Work out the finished part from the listing and answer in its coordinate system (mm). A direction names the side the tool comes from. Coordinates: 2 decimals unless noted, no trailing zeros. Write each loop counter-clockwise with the first axis right and the second up, starting at its lowest first coordinate (ties: lowest second). Pieces come first, ordered by that corner, then holes. Notation, with made-up numbers: (26.25, 10) - (72.25, 10) arc R20 ccw to (72.25, 20) - close; hole circle Ø4 at (60, -5.75). An arc over 180 degrees is marked (long way). One line per item, written item: value.
```python
from build123d import *

# Parameters (mm, degrees)
SKETCH1_R           = 17.35
BOSS_EXTRUDE1_DEPTH = 7
SKETCH2_R           = 31
BOSS_EXTRUDE2_DEPTH = 2
SKETCH3_R           = 14.646692659
CUT_EXTRUDE1_DEPTH  = 7
CHAMFER1_SIZE       = 1


with BuildPart() as part:
    # Sketch1 → Boss-Extrude1 (new body)
    with BuildSketch(Plane(origin=(0, 0, 0), x_dir=(1, 0, 0), z_dir=(0, 1, 0))):
        Circle(SKETCH1_R)
    extrude(amount=BOSS_EXTRUDE1_DEPTH)

    # Sketch2 → Boss-Extrude2 (add)
    with BuildSketch(Plane(origin=(0, 7, 0), x_dir=(1, 0, 0), z_dir=(0, 1, 0))):
        Circle(SKETCH2_R)
    extrude(amount=BOSS_EXTRUDE2_DEPTH)

    # Sketch3 → Cut-Extrude1 (cut)
    with BuildSketch(Plane.XZ):
        Circle(SKETCH3_R)
    extrude(amount=-CUT_EXTRUDE1_DEPTH, mode=Mode.SUBTRACT)

    # Chamfer1
    chamfer1_edges = [part.edges().sort_by_distance(p)[0] for p in [
        (-31, 9, 0),
    ]]
    chamfer(chamfer1_edges, length=CHAMFER1_SIZE)


solid = part.part
```
Item 1: Consider probe 1 along Z at (x, y) = (0, 4.5); probe 2 along Y at (x, z) = (-21.5, -7.5); probe 3 along Z at (x, y) = (7, 6). Determine where each line is inside the solid, lowest interval first.
Evaluation:
probe 1: z = -17.35 to -14.65, 14.65 to 17.35
probe 2: y = 7 to 9
probe 3: z = -15.88 to -12.87, 12.87 to 15.88
Item 2: Given pin 1 (3 mm diameter, centred on y = 6.5, z = 23.5, fed in from +X); pin 2 (23.5 mm diameter, centred on x = 0, z = 0, fed in from -Y); pin 3 (23.5 mm diameter, centred on x = -6.5, z = 2, fed in from -Y), each flat-ended and moving along its own axis, determine where each tip first touches the part or whether it passes through.
Evaluation:
pin 1: stops at x = 21.75
pin 2: stops at y = 7
pin 3: stops at y = 0
Item 3: Which of the six approach directions +Z, -Z, +X, -X, +Y, -Y give full straight-line access (tool end or side, diameter ignored) to faces 4 (the face through (13, 7, 13)), 5 (the face through (0, 9, 0))?
Evaluation:
face 4: -Y
face 5: +Z, -Z, +X, -X, +Y
Item 4: Determine the mould class of faces 1 (the face through (-2.259, 3.451, -17.202)), 2 (the face through (-12, 0, 9)), 3 (the face through (0, 7, 0)) for opening direction Z: +Z half, -Z half, draft (parallel to the pull), parting line (faces both ways), or undercut.
Evaluation:
face 1: parting line
face 2: draft
face 3: undercut
Item 5: Section B-B, the plane x = 0 is taken. Determine the outline of the cut face in (y, z), then the cut area to 3 significant figures.
Evaluation:
outline: (0, -17.35) - (7, -17.35) - (7, -31) - (8, -31) - (9, -30) - (9, 30) - (8, 31) - (7, 31) - (7, 17.35) - (0, 17.35) - (0, 14.65) - (7, 14.65) - (7, -14.65) - (0, -14.65) - close
area: 161 mm2
Item 6: Section A-A, the plane z = 0 is taken. Determine the outline of the cut face in (x, y), then the cut area to 3 significant figures.
Evaluation:
outline: (-31, 7) - (-17.35, 7) - (-17.35, 0) - (-14.65, 0) - (-14.65, 7) - (14.65, 7) - (14.65, 0) - (17.35, 0) - (17.35, 7) - (31, 7) - (31, 8) - (30, 9) - (-30, 9) - (-31, 8) - close
area: 161 mm2
Item 7: Section C-C, the plane y = 1.75 is taken. Determine the outline of the cut face in (x, z), then the cut area to 3 significant figures.
Evaluation:
outline: circle Ø34.7 at (0, 0); hole circle Ø29.29 at (0, 0)
area: 272 mm2
